Design review of the part built by this model. Coordinates are the model's own, in mm. Face numbers are marked on the shaded views. A direction names the side the tool comes from. Round coordinates to 2 decimals unless told otherwise and drop trailing zeros. Loops run counter-clockwise (first coordinate to the right, second up) from the corner with the lowest first, then second, coordinate; pieces in that order, holes last. Notation, with made-up numbers: (-29, 50.5) -> (-11, 50.5) arc R23 cw to (-11, 80.5) -> close; hole circle Ø2 at (40.25, 56). An arc over 180 degrees is marked (long way). Answer as CSV lines item,"result". Start each with the question number.
(1) Take a section at B-B, the plane y = 1.5. Write out the cut boundary in (x, z).
(2) Take a section at C-C, the plane z = 19. Write out the cut boundary in (x, y).
(3) Draft analysis for pull direction X (two halves, no side actions). For the marked faces 4, 5 and 6, state which applies: +X half, -X half, draft (parallel to the pull), parting line (faces both ways), or undercut.
(4) Take a section at A-A, the plane x = -51.5. Write out the cut boundary in (y, z), and give its area (3 significant figures).
(5) Take a section at D-D, the plane x = -32. Write out the cut boundary in (y, z).
(6) To check wall thickness, follow line 1 (Z direction, x = -50, y = 41); line 2 (X direction, y = 22.5, z = 9); line 3 (Y direction, x = -29.5, z = 8). State the ranges of each line that lie inside material, in increasing order. Write a range as from..to.
(7) Machinability: for the marked faces 1, 2 and 3, which of the approach directions +Z, -Z, +X, -X, +Y, -Y give a long, thin tool a straight path to every point of the face, cutting with its end or side? Answer none if there is none.
(8) For P1, Ø3, axis at x = -40.5, z = -0.5, coming from the -Y side; P2, Ø2, axis at x = -51.5, y = 31, coming from the +Z side; P3, Ø4, axis at x = -58.5, z = 11, coming from the -Y side, all flat-tipped, find the tip position at first contact; note any pin that passes through.
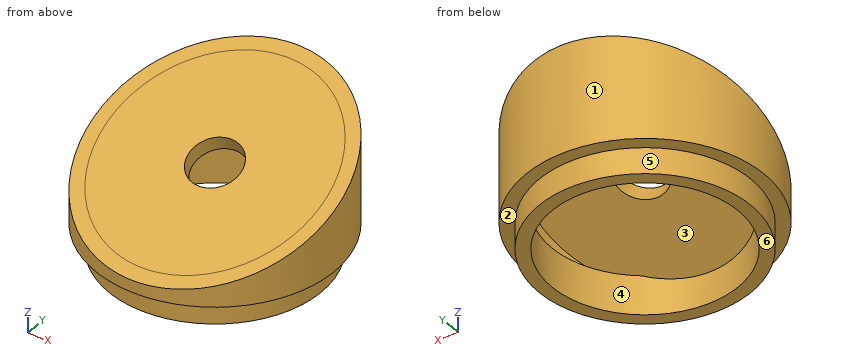
from build123d import *

# Parameters (mm, degrees)
F0_R      = 27.5
F0_R_2    = 24.5
F1_DEPTH  = 25
F3_DEPTH  = 82.3
F0_R_3    = 21.5
F7_DEPTH  = 3
F8_DEPTH  = 6
F9_R      = 5.9
F10_DEPTH = 12.8


with BuildPart() as f1:
    # F0 (on Top) → F1 (new body)
    with BuildSketch(Plane.XY):
        with Locations((-46.2939329445, 17.4860227853)):
            Circle(F0_R)
        with Locations((-46.2939329445, 17.4860227853)):
            Circle(F0_R_2, mode=Mode.SUBTRACT)
    extrude(amount=F1_DEPTH)

    # F2 (on Right) → F3 (cut)
    with BuildSketch(Plane.YZ):
        Polygon((44.9860227853, 25), (-10.0139772147, 25), (-10.0139772147, 2.7644119691), align=None)
    extrude(amount=-F3_DEPTH, mode=Mode.SUBTRACT)

    # F6: sweep along a path in F5
    with BuildLine(Plane.XZ) as f6_path:
        Line((-46.2939329445, 4.0015787818), (-46.2939329445, 0))
    # F4 (on face) → F6 (sweep)
    with BuildSketch(Plane(origin=(0, -2.3674011747, 5.8557958722), x_dir=(1, 0, 0), z_dir=(0, -0.3748115672, 0.9271010134))):
        with BuildLine():
            add(Edge.make_bspline(
                [(-21.7939329445, 21.4145208265), (-21.7939329445, -24.3574545801), (-58.5439329445, -1.4714668768), (-95.2939329445, 21.4145208265), (-58.5439329445, 44.3005085297), (-21.7939329445, 67.186496233), (-21.7939329445, 21.4145208265)],
                knots=[4.7123889804, 4.7123889804, 4.7123889804, 6.8067840828, 6.8067840828, 8.9011791852, 8.9011791852, 10.9955742876, 10.9955742876, 10.9955742876], degree=2, weights=[1, 0.5, 1, 0.5, 1, 0.5, 1]))
        make_face()
    sweep(path=f6_path.line)

    # F0 (on Top) → F7 (join)
    with BuildSketch(Plane.XY):
        with Locations((-46.2939329445, 17.4860227853)):
            Circle(F0_R_2)
        with Locations((-46.2939329445, 17.4860227853)):
            Circle(F0_R_3, mode=Mode.SUBTRACT)
    extrude(amount=F7_DEPTH)

    # F0 (on Top) → F8 (join)
    with BuildSketch(Plane.XY):
        with Locations((-46.2939329445, 17.4860227853)):
            Circle(F0_R_2)
        with Locations((-46.2939329445, 17.4860227853)):
            Circle(F0_R_3, mode=Mode.SUBTRACT)
    extrude(amount=-F8_DEPTH)

    # F9 (on face) → F10 (cut)
    with BuildSketch(Plane(origin=(0, -2.3674011747, 5.8557958722), x_dir=(1, 0, 0), z_dir=(0, -0.3748115672, 0.9271010134))):
        with Locations((-46.2939329445, 21.4145208265)):
            Circle(F9_R)
    extrude(amount=-F10_DEPTH, mode=Mode.SUBTRACT)


solid = f1.part
The answers:
1,outline,"(-68.67, 0) -> (-64.86, 0) -> (-64.86, -6) -> (-60.67, -6) -> (-60.67, 3) -> (-64.86, 3) -> (-64.86, 3.42) -> (-27.73, 3.42) -> (-27.73, 3) -> (-31.92, 3) -> (-31.92, -6) -> (-27.73, -6) -> (-27.73, 0) -> (-23.92, 0) -> (-23.92, 7.42) -> (-68.67, 7.42) -> close"
2,outline,"(-70.71, 30.14) -> (-21.88, 30.14) arc R27.5 ccw to start; hole (-55.86, 40.04) -> (-36.73, 40.04) arc R24.5 ccw to start"
3,face 4,"undercut"
3,face 5,"parting line"
3,face 6,"draft"
4,outline,"(-9.52, 0) -> (-6.45, 0) -> (-6.45, -6) -> (-3.37, -6) -> (-3.37, 1.45) -> (16.3, 9.4) -> (14.91, 12.84) -> (-9.52, 2.97) -> close; (20.06, 14.92) -> (21.45, 11.48) -> (41.43, 19.56) -> (41.43, 3) -> (38.35, 3) -> (38.35, -6) -> (41.43, -6) -> (41.43, 0) -> (44.49, 0) -> (44.49, 24.8) -> close"
4,area,"305 mm²"
5,outline,"(-6.01, 0) -> (-2.41, 0) -> (-2.41, -6) -> (1.43, -6) -> (1.43, 3) -> (0.47, 3) -> (37.38, 17.93) -> (37.38, 3) -> (33.55, 3) -> (33.55, -6) -> (37.38, -6) -> (37.38, 0) -> (40.98, 0) -> (40.98, 23.38) -> (-6.01, 4.38) -> close"
6,line 1,"-6..3, 19.39..23.39"
6,line 2,"-73.33..-70.28, -22.31..-19.25"
6,line 3,"2.94..12.83, 35.32..39.26"
7,face 1,"+Z, -Z"
7,face 2,"-Z"
7,face 3,"none"
8,P1,"y = -9.66"
8,P2,"z = 19.75"
8,P3,"y = 5.41"
